Can you work these out from the model? Positions are in its coordinate system, mm. A direction names the side the tool comes from. Coordinates: 2 decimals unless noted, no trailing zeros. Order: outer loops, then holes, each group sorted by start corner. A loop starts at its lowest first (then second) coordinate and runs counter-clockwise, first axis right, second up. Notation, with made-up numbers: (28, 83) -> (37, 83) arc R20 ccw to (37, 95) -> close; hole circle Ø9 at (44.5, -26.75). An arc over 180 degrees is marked (long way). Answer in a Markdown table with one row per item. Add a question column.
1. Imagine slicing it at D-D on y = -6.5. Write out the boundary of the cut face in (x, z).
2. If I drill on line 1 along Y through (x, z) = (-12.6, 0); line 2 along Y through (x, z) = (-7, 0); line 3 along X through (y, z) = (0, -19), over which ranges is the centre line in solid material (lowest first)? Write a range as [from, to].
3. Imagine slicing it at C-C on x = -4.5. Write out the boundary of the cut face in (y, z).
4. We'd pull the mould along Y, two halves only. Please class faces 1 (the face through (-15, 0, -10)), 2 (the face through (-12.288, -7.907, -1.756)), 3 (the face through (-8.409, -19.961, -10.382)): pulls with the +Y half, pulls with the -Y half, needs draft (parallel to the pull), parting line crosses it, or undercut.
5. Will these pins go through, and if not, where does the flat tip stop? pin 1 (3 mm diameter, centred on x = -11.5, z = 0, fed in from +Y); pin 2 (2 mm diameter, centred on x = -6.5, z = 16.5, fed in from -Y); pin 3 (3 mm diameter, centred on x = -8.5, y = -4, fed in from -Z).
6. On a 3-axis mill with a long thin cutter (end or side, diameter ignored), from which of +Z, -Z, +X, -X, +Y, -Y can I reach the whole of each face in a straight line? I mean faces 4 (the face through (-9.5, 0, 3)), 5 (the face through (-4.684, -2.685, 0.596)), 6 (the face through (-0.986, 3.755, -11.923)). Say none if no direction works.
7. Imagine slicing it at A-A on y = 0. Write out the boundary of the cut face in (x, z).
from build123d import *

# Parameters (mm, degrees)
SKETCH1_R               = 22.5
BOSS_EXTRUDE1_DEPTH     = 15
SKETCH2_R               = 2.75
CUT_EXTRUDE1_DEPTH      = 36.178118199
SKETCH5_R               = 8.1
CUT_EXTRUDE2_DEPTH      = 5.5
SKETCH28_R              = 22.5
SKETCH28_R_2            = 12.5
CUT_EXTRUDE_THIN1_DEPTH = 2


with BuildPart() as part:
    # Sketch1 → Boss-Extrude1 (new body)
    with BuildSketch(Plane(origin=(0, 0, 0), x_dir=(0, 0, -1), z_dir=(1, 0, 0))):
        Circle(SKETCH1_R)
    extrude(amount=-BOSS_EXTRUDE1_DEPTH)

    # Sketch2 → Cut-Extrude1 (cut, through all)
    with BuildSketch(Plane(origin=(0, 0, 0), x_dir=(0, 0, -1), z_dir=(1, 0, 0))):
        Circle(SKETCH2_R)
    extrude(amount=-CUT_EXTRUDE1_DEPTH, mode=Mode.SUBTRACT)

    # Sketch5 → Cut-Extrude2 (cut)
    with BuildSketch(Plane.ZY.offset(15)):
        Circle(SKETCH5_R)
    extrude(amount=-CUT_EXTRUDE2_DEPTH, mode=Mode.SUBTRACT)

    # Sketch28 → Cut-Extrude-Thin1 (cut)
    with BuildSketch(Plane(origin=(0, 0, 0), x_dir=(0, 0, -1), z_dir=(1, 0, 0))):
        Circle(SKETCH28_R)
        Circle(SKETCH28_R_2, mode=Mode.SUBTRACT)
    extrude(amount=-CUT_EXTRUDE_THIN1_DEPTH, mode=Mode.SUBTRACT)


solid = part.part
Answers follow:
| question | item | result |
|---|---|---|
| 1 | outline | (-15, -21.54) -> (-2, -21.54) -> (-2, -10.68) -> (0, -10.68) -> (0, 10.68) -> (-2, 10.68) -> (-2, 21.54) -> (-15, 21.54) -> (-15, 4.83) -> (-9.5, 4.83) -> (-9.5, -4.83) -> (-15, -4.83) -> close |
| 2 | line 1 | y = [-22.5, -8.1], [8.1, 22.5] |
| 2 | line 2 | y = [-22.5, -2.75], [2.75, 22.5] |
| 2 | line 3 | x = [-15, -2] |
| 3 | outline | circle Ø45 at (0, 0); hole circle Ø5.5 at (0, 0) |
| 4 | face 1 | needs draft |
| 4 | face 2 | undercut |
| 4 | face 3 | parting line crosses it |
| 5 | pin 1 | stops at y = 22.5 |
| 5 | pin 2 | stops at y = -16.31 |
| 5 | pin 3 | stops at z = -22.36 |
| 6 | face 4 | -X |
| 6 | face 5 | +X, -X |
| 6 | face 6 | +X |
| 7 | outline | (-15, -22.5) -> (-2, -22.5) -> (-2, -12.5) -> (0, -12.5) -> (0, -2.75) -> (-9.5, -2.75) -> (-9.5, -8.1) -> (-15, -8.1) -> close; (-15, 8.1) -> (-9.5, 8.1) -> (-9.5, 2.75) -> (0, 2.75) -> (0, 12.5) -> (-2, 12.5) -> (-2, 22.5) -> (-15, 22.5) -> close |
